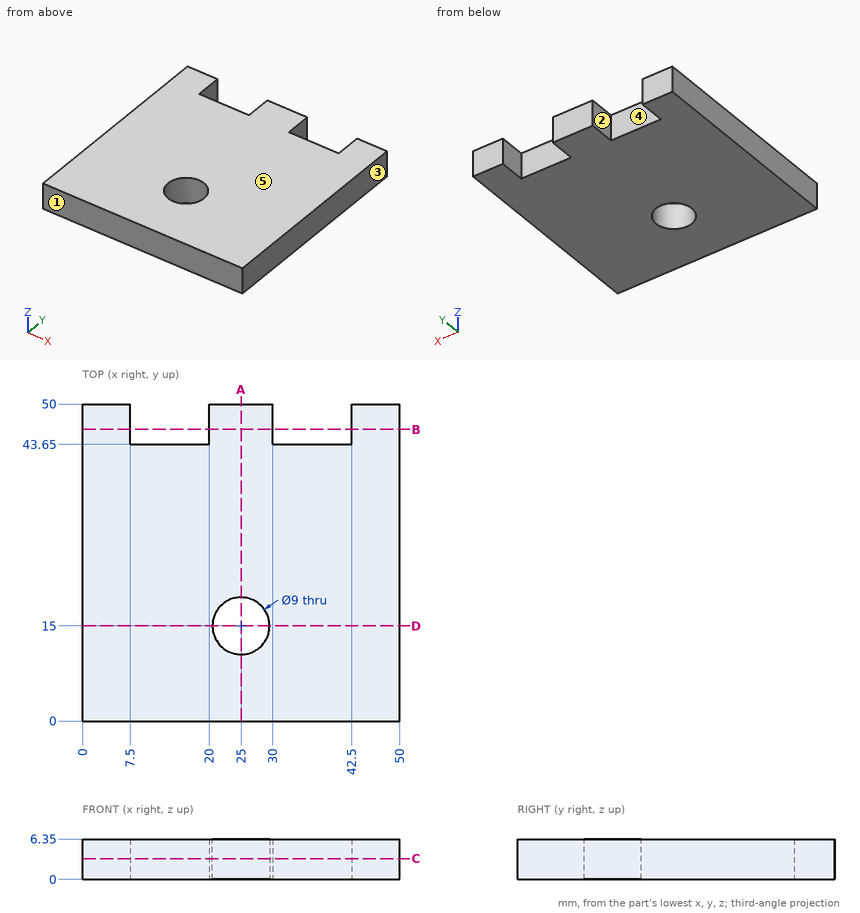
Source: three-view drawing plus pictorial views. Frame: mm from the lowest corner of the part. A direction names the side the tool comes from. Round coordinates to 2 decimals unless told otherwise and drop trailing zeros. Loops run counter-clockwise (first coordinate to the right, second up) from the corner with the lowest first, then second, coordinate; pieces in that order, holes last. Notation, with made-up numbers: M 37.5,40.25 L 70.5,40.25 A15 ccw 70.5,57.25 Z; hole C 11.5,6.25 d2. An arc over 180 degrees is marked long. Answer as CSV lines item,"result". Start each with the question number.
(1) Section A-A, the plane x = 25. Output: boundary loops of the cut face in (y, z).
(2) Draft query along X for the marked faces 3, 4 and 5. Return one class per face: released by +X, released by -X, zero draft, split by the parting line, or undercut.
(3) First-contact query: pin 1 (3 mm diameter, centred on x = 38, z = 2, fed in from +Y). Flat tip, straight axial feed; report the tip coordinate or a pass-through.
(4) Reachability of the marked faces 1 and 2 from +Z, -Z, +X, -X, +Y, -Y: full face, straight path, thin tool, end or side. Return the list, or none.
(5) Section B-B, the plane y = 46. Output: boundary loops of the cut face in (x, z), plus the area to 3 significant figures.
(6) Line query: line 1 (X direction, y = 47.5, z = 2); line 2 (Y direction, x = 25, z = 2.75); line 3 (Y direction, x = 17, z = 6). Output: solid intervals per line, ascending. Write a range as [from, to].
(7) Section C-C, the plane z = 3.25. Output: boundary loops of the cut face in (x, y), plus the area to 3 significant figures.
(8) Section D-D, the plane y = 15. Output: boundary loops of the cut face in (x, z).
Values found:
1,outline,"M 0,0 L 10.5,0 L 10.5,6.35 L 0,6.35 Z; M 19.5,0 L 50,0 L 50,6.35 L 19.5,6.35 Z"
2,face 3,"released by +X"
2,face 4,"undercut"
2,face 5,"zero draft"
3,pin 1,"stops at y = 43.65"
4,face 1,"+Z, -Z, +X, -X, -Y"
4,face 2,"+Z, -Z, +Y"
5,outline,"M 0,0 L 7.5,0 L 7.5,6.35 L 0,6.35 Z; M 20,0 L 30,0 L 30,6.35 L 20,6.35 Z; M 42.5,0 L 50,0 L 50,6.35 L 42.5,6.35 Z"
5,area,"159 mm²"
6,line 1,"x = [0, 7.5], [20, 30], [42.5, 50]"
6,line 2,"y = [0, 10.5], [19.5, 50]"
6,line 3,"y = [0, 43.65]"
7,outline,"M 0,0 L 50,0 L 50,50 L 42.5,50 L 42.5,43.65 L 30,43.65 L 30,50 L 20,50 L 20,43.65 L 7.5,43.65 L 7.5,50 L 0,50 Z; hole C 25,15 d9"
7,area,"2,280 mm²"
8,outline,"M 0,0 L 20.5,0 L 20.5,6.35 L 0,6.35 Z; M 29.5,0 L 50,0 L 50,6.35 L 29.5,6.35 Z"
